The figure shows three views and two pictorial views of one solid part (mm, origin at its lowest corner). Answer the questions. Coordinates: 2 decimals unless noted, no trailing zeros. Order: outer loops, then holes, each group sorted by start corner. A loop starts at its lowest first (then second) coordinate and runs counter-clockwise, first axis right, second up. Notation, with made-up numbers: (-20, 52.5) -> (35, 52.5) arc R31 cw to (35, 84.5) -> close; hole circle Ø1 at (52, -30.75). An arc over 180 degrees is marked (long way). Write item = value, one per line. Start each with the question number.
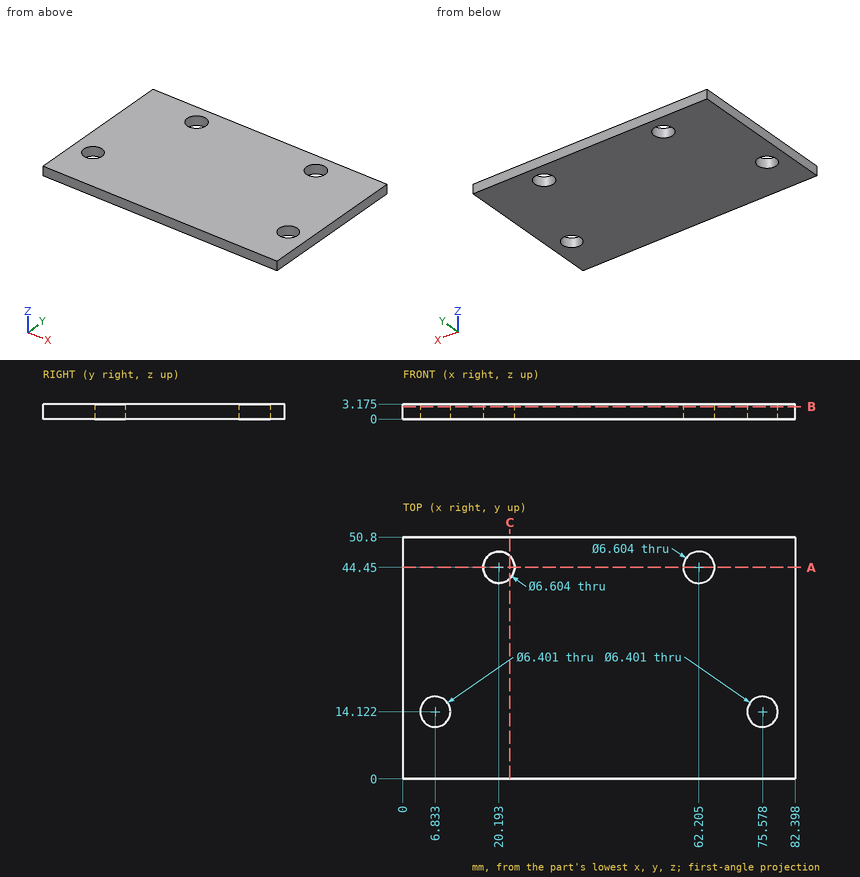
Item 1: Section C-C, the plane x = 22.5 is taken. Give the vertices of the cut face in (y, z) (1 decimal).
Item 2: Section B-B, the plane z = 2.6 is taken. Give the number of separate pieces and of enclosed holes in the cut face, then the cut area to 3 significant figures.
Item 3: Consider probe 1 along X at (y, z) = (45, 1.3); probe 2 along X at (y, z) = (42.5, 0.45); probe 3 along Y at (x, z) = (20, 2.35). Determine where each line is inside the solid, lowest interval first.
Item 4: This flat-tipped pin is pushed along its axis until it touches: pin 1 (10 mm diameter, centred on x = 75.58, y = 14.12, fed in from +Z) (3 decimals). Where does it stop, or does it pass through?
Item 5: Section A-A, the plane y = 44.45 is taken. Give the vertices of the cut face in (x, z) (1 decimal).
A:
q1.outline = (0, 0) -> (42.1, 0) -> (42.1, 3.2) -> (0, 3.2) -> close; (46.8, 0) -> (50.8, 0) -> (50.8, 3.2) -> (46.8, 3.2) -> close
q2.separate_pieces = 1
q2.enclosed_holes = 4
q2.area = 4,050 mm^2
q3.probe_1 = 0 to 16.94, 23.45 to 58.95, 65.46 to 82.4
q3.probe_2 = 0 to 17.53, 22.86 to 59.54, 64.87 to 82.4
q3.probe_3 = 0 to 41.15, 47.75 to 50.8
q4.pin_1 = 3.175
q5.outline = (0, 0) -> (16.9, 0) -> (16.9, 3.2) -> (0, 3.2) -> close; (23.5, 0) -> (58.9, 0) -> (58.9, 3.2) -> (23.5, 3.2) -> close; (65.5, 0) -> (82.4, 0) -> (82.4, 3.2) -> (65.5, 3.2) -> close
